```python
from build123d import *

# Parameters (mm, degrees)
F0_R     = 8
F1_DEPTH = 26
F2_R     = 12
F2_R_2   = 1.7
F3_DEPTH = 25
F5_DEPTH = 20.001


# Not quite as in the source:
# - a pattern or mirror of a feature is missing from the dataset's text; its kind, count and spacing are read off the source's solid


with BuildPart() as f1:
    # F0 (on Right) → F1 (new body, symmetric)
    with BuildSketch(Plane.YZ):
        with BuildLine():
            ThreePointArc((2, 29), (19.4868329805, 38.1622776602), (0, 35))
            Line((0, 35), (0, -35))
            ThreePointArc((0, -35), (19.4868329805, -38.1622776602), (2, -29))
            Line((2, -29), (2, 29))
        make_face()
        with Locations((10, -35)):
            Circle(F0_R, mode=Mode.SUBTRACT)
        with Locations((10, 35)):
            Circle(F0_R, mode=Mode.SUBTRACT)
    extrude(amount=F1_DEPTH, both=True)

    # F2 (on face) → F3 (cut)
    with BuildSketch(Plane.XZ):
        Circle(F2_R)
        with Locations((-15.5, 15.5)):
            Circle(F2_R_2)
        with Locations((15.5, 15.5)):
            Circle(F2_R_2)
        with Locations((15.5, -15.5)):
            Circle(F2_R_2)
        with Locations((-15.5, -15.5)):
            Circle(F2_R_2)
    extrude(amount=-F3_DEPTH, mode=Mode.SUBTRACT)

    # F4 (on face) → F5 (cut, through all)
    with BuildSketch(Plane.XZ):
        with BuildLine():
            Line((1, 19.4743420942), (1, 45))
            Line((1, 45), (-1, 45))
            Line((-1, 45), (-1, 19.4743420942))
            ThreePointArc((-1, 19.4743420942), (0, 19.5), (1, 19.4743420942))
        make_face()
    f5 = extrude(amount=-F5_DEPTH, mode=Mode.SUBTRACT)

    # F5_copies: F5 across plane
    add(f5.mirror(Plane(origin=(0, 0, 0), x_dir=(-1, 0, 0), z_dir=(0, 0, -1))), mode=Mode.SUBTRACT)


solid = f1.part
```
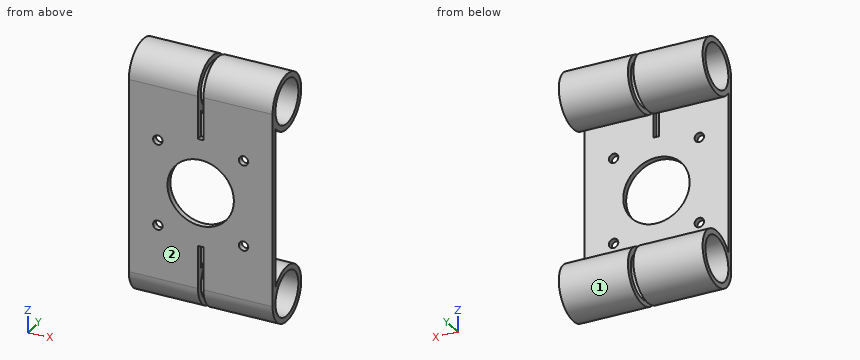
Geometry: final body of the model. Coordinates: model frame, mm. Face numbers are marked on the shaded views. Round coordinates to 2 decimals unless told otherwise and drop trailing zeros. Write each loop counter-clockwise with the first axis right and the second up, starting at its lowest first coordinate (ties: lowest second). Pieces come first, ordered by that corner, then holes. Notation, with made-up numbers: M 62.25,51 L 94.25,51 A18 cw 94.25,61 Z; hole C 21.5,15.25 d4. An arc over 180 degrees is marked long. Answer in a Markdown table with one row per item. Add a question column.
(1) Cut plane A-A, the plane z = 0. Return the cut outline in (x, y).
(2) Cut plane C-C, the plane y = 10. Give the number of separate pieces and of enclosed holes in the cut face, then the cut area to 3 significant figures.
(3) Ray query, L1, parallel to Z at x = -10.5, y = 10; L2, parallel to Y at x = 16.75, z = -35; L3, parallel to X at y = 6, z = -26. Return the intervals inside material, ascending.
(4) Draft query along Z for the marked faces 1 and 2. Return one class per face: pulls with the +Z half, pulls with the -Z half, needs draft (parallel to the pull), parting line crosses it, or undercut.
(5) Cut plane D-D, the plane x = 2. Return the cut outline in (y, z), then the cut area to 3 significant figures.
(6) Contact query for flat-ended pins moving along their axis: pin 1 (4.5 mm diameter, centred on x = -15.5, z = 15.5, fed in from -Y); pin 2 (5 mm diameter, centred on x = -15.5, y = 5, fed in from +Z); pin 3 (8 mm diameter, centred on x = -14.5, z = 23.5, fed in from +Y); pin 4 (5.5 mm diameter, centred on x = -15.5, z = -15.5, fed in from +Y). Output: stop coordinate, or through.
(7) Cut plane B-B, the plane x = 15.5. Return the cut outline in (y, z), then the cut area to 3 significant figures.
Established:
| question | item | result |
|---|---|---|
| 1 | outline | M -26,0 L -12,0 L -12,2 L -26,2 Z; M 12,0 L 26,0 L 26,2 L 12,2 Z |
| 2 | separate pieces | 8 |
| 2 | enclosed holes | 0 |
| 2 | area | 400 mm² |
| 3 | L1 | -45 to -43, -27 to -25, 25 to 27, 43 to 45 |
| 3 | L2 | 0 to 2, 18 to 20 |
| 3 | L3 | -26 to -1, 1 to 26 |
| 4 | face 1 | undercut |
| 4 | face 2 | needs draft |
| 5 | outline | M 0,-35 A10 ccw long 2,-29 L 2,-11.83 L 0,-11.83 Z; M 0,11.83 L 2,11.83 L 2,29 A10 ccw long 0,35 Z; hole C 10,-35 d16; hole C 10,35 d16 |
| 5 | area | 303 mm² |
| 6 | pin 1 | y = 0 |
| 6 | pin 2 | z = 44.68 |
| 6 | pin 3 | y = 16.61 |
| 6 | pin 4 | y = 2 |
| 7 | outline | M 0,-35 A10 ccw long 2,-29 L 2,-17.2 L 0,-17.2 Z; M 0,-13.8 L 2,-13.8 L 2,13.8 L 0,13.8 Z; M 0,17.2 L 2,17.2 L 2,29 A10 ccw long 0,35 Z; hole C 10,-35 d16; hole C 10,35 d16 |
| 7 | area | 336 mm² |
